The model under review builds one solid part; all positions refer to its coordinate system, in mm. Face numbers are marked on the shaded views. A direction names the side the tool comes from. Round coordinates to 2 decimals unless told otherwise and drop trailing zeros. Write each loop counter-clockwise with the first axis right and the second up, starting at its lowest first coordinate (ties: lowest second). Pieces come first, ordered by that corner, then holes. Notation, with made-up numbers: (2, 0.5) - (48, 0.5) arc R11 ccw to (48, 17.5) - close; hole circle Ø4 at (-19, 56.5). An arc over 180 degrees is marked (long way). Return JSON: item names as keys, results as strings.
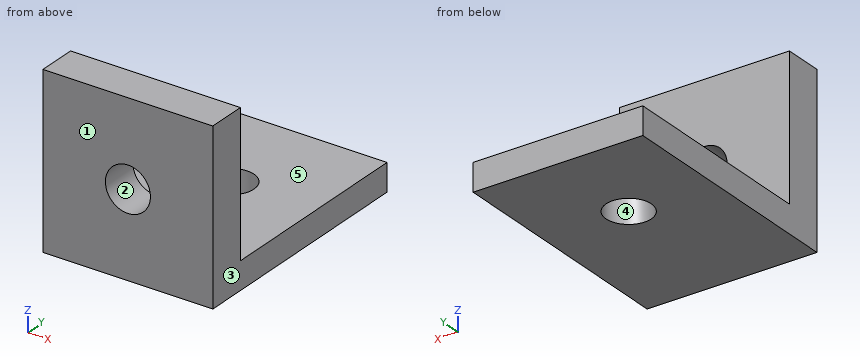
from build123d import *

# Parameters (mm, degrees)
SKETCH1_W           = 20
SKETCH1_H           = 20
SKETCH1_R           = 2.65
BOSS_EXTRUDE1_DEPTH = 4.6
SKETCH2_W           = 20
SKETCH2_H           = 3.25
BOSS_EXTRUDE2_DEPTH = 24.5
SKETCH3_R           = 2.665
CUT_EXTRUDE1_DEPTH  = 37.698910066


with BuildPart() as part:
    # Sketch1 → Boss-Extrude1 (new body)
    with BuildSketch(Plane(origin=(0, 0, 0), x_dir=(1, 0, 0), z_dir=(0, 1, 0))):
        Rectangle(SKETCH1_W, SKETCH1_H)
        with Locations(Location((0, 0, 0), (0, 0, 270))):
            Circle(SKETCH1_R, mode=Mode.SUBTRACT)
    extrude(amount=BOSS_EXTRUDE1_DEPTH)

    # Sketch2 → Boss-Extrude2 (add)
    with BuildSketch(Plane(origin=(0, 4.6, 0), x_dir=(1, 0, 0), z_dir=(0, 1, 0))):
        with Locations((0, 8.375)):
            Rectangle(SKETCH2_W, SKETCH2_H)
    extrude(amount=BOSS_EXTRUDE2_DEPTH)

    # Sketch3 → Cut-Extrude1 (cut, through all)
    with BuildSketch(Plane(origin=(0, 0, -10), x_dir=(-1, 0, 0), z_dir=(0, 0, -1))):
        with Locations((0, 17.275)):
            Circle(SKETCH3_R)
    extrude(amount=-CUT_EXTRUDE1_DEPTH, mode=Mode.SUBTRACT)


solid = part.part
(1) Add section A-A (z = 0). Write out the cut boundary in (x, y), plus the area to 3 significant figures.
Filled in:
{"outline": "(-10, 0) - (-2.65, 0) - (-2.65, 4.6) - (-10, 4.6) - close; (2.65, 0) - (10, 0) - (10, 4.6) - (2.65, 4.6) - close", "area": "67.6 mm2"}
(2) Add section B-B (x = 0). Write out the cut boundary in (y, z), plus the area to 3 significant figures.
Filled in:
{"outline": "(0, -10) - (14.61, -10) - (14.61, -6.75) - (4.6, -6.75) - (4.6, -2.65) - (0, -2.65) - close; (0, 2.65) - (4.6, 2.65) - (4.6, 10) - (0, 10) - close; (19.94, -10) - (29.1, -10) - (29.1, -6.75) - (19.94, -6.75) - close", "area": "130 mm2"}
(3) Wall thickness on line 1 (Y direction, x = 0, z = -8.8); line 2 (X direction, y = 3.35, z = 0); line 3 (Z direction, x = 9, y = 6.75): over which ranges is each line inside the solid? List them lowest first.
Filled in:
{"line 1": "y = 0 to 14.61, 19.94 to 29.1", "line 2": "x = -10 to -2.65, 2.65 to 10", "line 3": "z = -10 to -6.75"}
(4) Mouldability with a two-part tool opening along X and no side actions: class the marked faces 1, 2 and 3 as released by +X, released by -X, zero draft, split by the parting line, or undercut.
Filled in:
{"face 1": "zero draft", "face 2": "undercut", "face 3": "released by +X"}
(5) Clearance check with flat-ended pins moving along their axes: pin 1 Ø2 at (x, z) = (1, 4) entering from +Y; pin 2 Ø6 at (x, y) = (1, 21.5) entering from +Z. State where each tip first meets the part, or that it passes through.
Filled in:
{"pin 1": "stops at y = 4.6", "pin 2": "stops at z = -6.75"}
(6) For the marked faces 4 and 5, list the 3-axis set-ups (+Z, -Z, +X, -X, +Y, -Y) from which the entire face can be reached by the end or side of a thin tool; tool diameter is ignored.
Filled in:
{"face 4": "+Z, -Z", "face 5": "+Z, +X, -X, +Y"}
(7) Add section D-D (y = 18.5). Write out the cut boundary in (x, z).
Filled in:
{"outline": "(-10, -10) - (-2.37, -10) - (-2.37, -6.75) - (-10, -6.75) - close; (2.37, -10) - (10, -10) - (10, -6.75) - (2.37, -6.75) - close"}
(8) Add section C-C (y = 2). Write out the cut boundary in (x, z).
Filled in:
{"outline": "(-10, -10) - (10, -10) - (10, 10) - (-10, 10) - close; hole circle Ø5.3 at (0, 0)"}
